Design review of the part shown in the three views and the two pictorial views. Dimensions are in mm from the part's minimum x, y and z. A direction names the side the tool comes from. Round coordinates to 2 decimals unless told otherwise and drop trailing zeros. Order: outer loops, then holes, each group sorted by start corner. A loop starts at its lowest first (then second) coordinate and runs counter-clockwise, first axis right, second up. Notation, with made-up numbers: (13, 15) - (69, 15) arc R20 ccw to (69, 22) - close; hole circle Ø5 at (33, 69.5). An arc over 180 degrees is marked (long way). One line per item, written item: value.
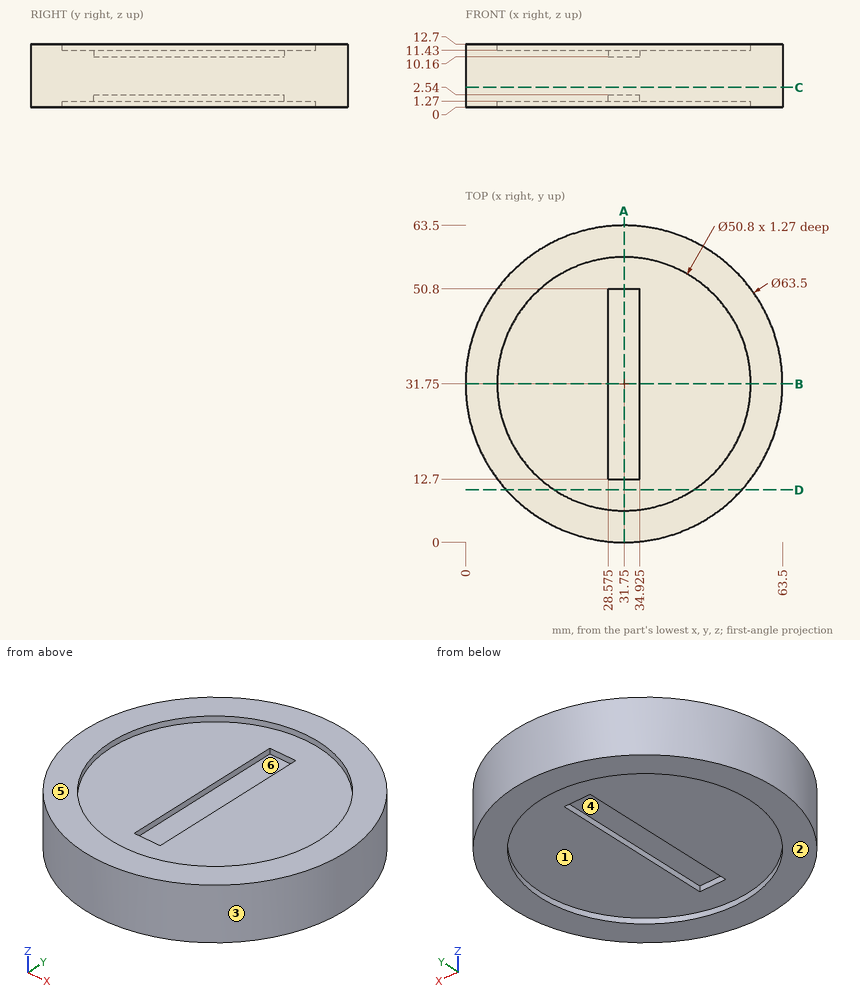
Item 1: For P1, Ø6, axis at x = 40.5, z = 3, coming from the +Y side (3 decimals); P2, Ø1.9, axis at x = 31.5, y = 29.5, coming from the +Z side; P3, Ø3, axis at x = 15.5, z = 10.5, coming from the -Y side, all flat-tipped, find the tip position at first contact; note any pin that passes through.
Returned:
P1: y = 62.975
P2: z = 10.16
P3: y = 3.63
Item 2: The part is to be moulded in two halves that separate along Y. For the marked faces 1, 2, 3 and 4, say which applies: +Y half, -Y half, draft (parallel to the pull), parting line (faces both ways), or undercut.
Returned:
face 1: undercut
face 2: draft
face 3: parting line
face 4: undercut
Item 3: Take a section at C-C (z = 4). Write out the cut boundary in (x, y), plus the area to 3 significant figures.
Returned:
outline: circle Ø63.5 at (31.75, 31.75)
area: 3,170 mm^2
Item 4: Take a section at B-B (y = 31.75). Write out the cut boundary in (x, z) (3 decimals), plus the area to 3 significant figures.
Returned:
outline: (0, 0) - (6.35, 0) - (6.35, 1.27) - (28.575, 1.27) - (28.575, 2.54) - (34.925, 2.54) - (34.925, 1.27) - (57.15, 1.27) - (57.15, 0) - (63.5, 0) - (63.5, 12.7) - (57.15, 12.7) - (57.15, 11.43) - (34.925, 11.43) - (34.925, 10.16) - (28.575, 10.16) - (28.575, 11.43) - (6.35, 11.43) - (6.35, 12.7) - (0, 12.7) - close
area: 661 mm^2
Item 5: Take a section at D-D (y = 10.5). Write out the cut boundary in (x, z), plus the area to 3 significant figures.
Returned:
outline: (8.16, 0) - (17.84, 0) - (17.84, 1.27) - (45.66, 1.27) - (45.66, 0) - (55.34, 0) - (55.34, 12.7) - (45.66, 12.7) - (45.66, 11.43) - (17.84, 11.43) - (17.84, 12.7) - (8.16, 12.7) - close
area: 529 mm^2
Item 6: Machinability: for the marked faces 5 and 6, which of the approach directions +Z, -Z, +X, -X, +Y, -Y give a long, thin tool a straight path to every point of the face, cutting with its end or side? Answer none if there is none.
Returned:
face 5: +Z, +X, -X, +Y, -Y
face 6: +Z
Item 7: Wall thickness on line 1 (Y direction, x = 31.75, z = 0.5); line 2 (Z direction, x = 40, y = 20); line 3 (X direction, y = 48, z = 0.5): over which ranges is each line inside the solid? List them lowest first.
Returned:
line 1: 0 to 6.35, 57.15 to 63.5
line 2: 1.27 to 11.43
line 3: 4.47 to 12.23, 51.27 to 59.03
Item 8: Take a section at A-A (x = 31.75). Write out the cut boundary in (y, z), plus the area to 3 significant figures.
Returned:
outline: (0, 0) - (6.35, 0) - (6.35, 1.27) - (12.7, 1.27) - (12.7, 2.54) - (50.8, 2.54) - (50.8, 1.27) - (57.15, 1.27) - (57.15, 0) - (63.5, 0) - (63.5, 12.7) - (57.15, 12.7) - (57.15, 11.43) - (50.8, 11.43) - (50.8, 10.16) - (12.7, 10.16) - (12.7, 11.43) - (6.35, 11.43) - (6.35, 12.7) - (0, 12.7) - close
area: 581 mm^2
